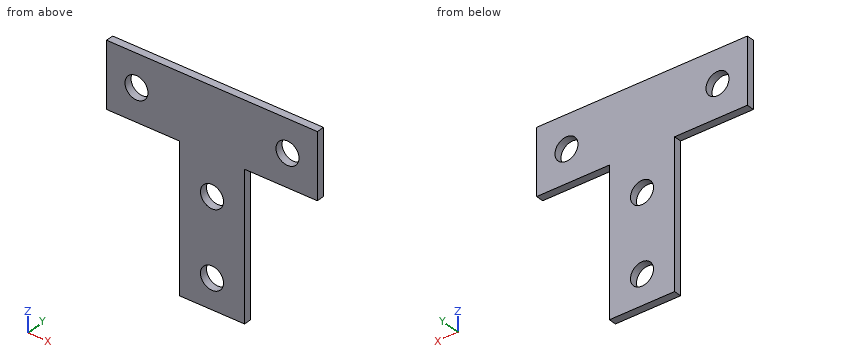
from build123d import *

# Parameters (mm, degrees)
SKETCH_1_W          = 55
SKETCH_1_H          = 55
EXTRUDE_1_DEPTH     = 2
SKETCH_2_W          = 19
SKETCH_2_H          = 38
CUT_EXTRUDE_1_DEPTH = 39.942264957
SKETCH_3_R          = 3
CUT_EXTRUDE_2_DEPTH = 39.942264957


with BuildPart() as part:
    # 草图1 → 凸台-拉伸1 (new body)
    with BuildSketch(Plane(origin=(0, 0, 0), x_dir=(1, 0, 0), z_dir=(0, 1, 0))):
        Rectangle(SKETCH_1_W, SKETCH_1_H)
    extrude(amount=EXTRUDE_1_DEPTH)

    # 草图2 → 切除-拉伸1 (cut, through all)
    with BuildSketch(Plane(origin=(0, 2, 0), x_dir=(1, 0, 0), z_dir=(0, 1, 0))):
        with Locations((-18, 8.5)):
            Rectangle(SKETCH_2_W, SKETCH_2_H)
        with Locations((18, 8.5)):
            Rectangle(SKETCH_2_W, SKETCH_2_H)
    extrude(amount=-CUT_EXTRUDE_1_DEPTH, mode=Mode.SUBTRACT)

    # 草图3 → 切除-拉伸2 (cut, through all)
    with BuildSketch(Plane(origin=(0, 2, 0), x_dir=(1, 0, 0), z_dir=(0, 1, 0))):
        with Locations(Location((-19.7, -19, 0), (0, 0, 270))):
            Circle(SKETCH_3_R)
        with Locations(Location((19.7, -19, 0), (0, 0, 270))):
            Circle(SKETCH_3_R)
        with Locations(Location((0, -0.3, 0), (0, 0, 270))):
            Circle(SKETCH_3_R)
        with Locations(Location((0, 19.7, 0), (0, 0, 270))):
            Circle(SKETCH_3_R)
    extrude(amount=-CUT_EXTRUDE_2_DEPTH, mode=Mode.SUBTRACT)


solid = part.part
Can you work these out from the model? Positions are in its coordinate system, mm. Coordinates: 2 decimals unless noted, no trailing zeros. Loops run counter-clockwise (first coordinate to the right, second up) from the corner with the lowest first, then second, coordinate; pieces in that order, holes last. Notation, with made-up numbers: M -40,88.25 L -33,88.25 A19 cw -33,92.25 Z; hole C 9,-9 d1. An arc over 180 degrees is marked long. Return JSON: item names as keys, results as strings. Group by question number.
Item 1: If I drill on L1, parallel to X at y = 0.6, z = 19; L2, parallel to X at y = 1.25, z = -19.7; L3, parallel to X at y = 1.3, z = -13, over which ranges is the centre line in solid material (lowest first)? Write a range as from..to.
Item 2: Imagine slicing it at A-A (z = 19). Please give me the cut outline in (x, y), and give its area (3 significant figures).
Item 3: I'm going to push a flat-ended pin straight in: pin 1 Ø3.5 at (x, z) = (19.7, 19) entering from -Y. Where does the tip first touch, or does it pass through?
Item 4: Imagine slicing it at C-C (x = 19.7). Please give me the cut outline in (y, z).
Item 5: Imagine slicing it at B-B (x = 0). Please give me the cut outline in (y, z).
Item 6: Imagine slicing it at D-D (y = 0.3). Please give me the cut outline in (x, z), and give its area (3 significant figures).
Verdict:
{
 "1": {"L1": "x = -27.5..-22.7, -16.7..16.7, 22.7..27.5", "L2": "x = -8.5..-3, 3..8.5", "L3": "x = -8.5..8.5"},
 "2": {"outline": "M -27.5,0 L -22.7,0 L -22.7,2 L -27.5,2 Z; M -16.7,0 L 16.7,0 L 16.7,2 L -16.7,2 Z; M 22.7,0 L 27.5,0 L 27.5,2 L 22.7,2 Z", "area": "86.0 mm^2"},
 "3": {"pin 1": "passes through"},
 "4": {"outline": "M 0,10.5 L 2,10.5 L 2,16 L 0,16 Z; M 0,22 L 2,22 L 2,27.5 L 0,27.5 Z"},
 "5": {"outline": "M 0,-27.5 L 2,-27.5 L 2,-22.7 L 0,-22.7 Z; M 0,-16.7 L 2,-16.7 L 2,-2.7 L 0,-2.7 Z; M 0,3.3 L 2,3.3 L 2,27.5 L 0,27.5 Z"},
 "6": {"outline": "M -27.5,10.5 L -8.5,10.5 L -8.5,-27.5 L 8.5,-27.5 L 8.5,10.5 L 27.5,10.5 L 27.5,27.5 L -27.5,27.5 Z; hole C -19.7,19 d6; hole C 0,-19.7 d6; hole C 0,0.3 d6; hole C 19.7,19 d6", "area": "1,470 mm^2"}
}
